from build123d import *

# Parameters (mm, degrees)
BASE_FLANGE1_DEPTH           = 50.8
CUT_EXTRUDE1_DEPTH           = 72.510156621
CUT_EXTRUDE1_DEPTH_BACK      = 72.510156621
SKETCH6_W                    = 21.9
SKETCH6_H                    = 58.896012785
SKETCH6_W_2                  = 19
F_7_0_7_DIAMETER_HOLE1_D     = 7
F_7_0_7_DIAMETER_HOLE1_DEPTH = 10
F_7_0_7_DIAMETER_HOLE1_TIP   = 2.103012167
CUT_EXTRUDE2_DEPTH           = 10
CHAMFER1_SIZE                = 0.5


# Sheet-metal steps are written as plain solids
with BuildPart() as part:
    # Sketch1 → Base-Flange1 (new, symmetric)
    with BuildSketch(Plane(origin=(0, 0, 0), x_dir=(0, 0, -1), z_dir=(1, 0, 0))):
        with BuildLine():
            Line((50, -4.5), (5.275314915, -4.5))
            ThreePointArc((5.275314915, -4.5), (3.603327521, -4.640767872), (1.978412548, -5.059108369))
            Line((1.978412548, -5.059108369), (0.835379329, -5.458272884))
            ThreePointArc((0.835379329, -5.458272884), (-0.371159142, -5.680341687), (-1.588253888, -5.526296191))
            ThreePointArc((-1.588253888, -5.526296191), (-2.687165368, 5.083467546), (5.460998077, -1.8))
            Line((5.460998077, -1.8), (3.086651087, -1.017391304))
            ThreePointArc((3.086651087, -1.017391304), (-1.518832599, 2.873264265), (-0.897708719, -3.123558716))
            ThreePointArc((-0.897708719, -3.123558716), (-0.44129819, -3.181325777), (0.011153737, -3.098049977))
            Line((0.011153737, -3.098049977), (1.154186957, -2.698885462))
            ThreePointArc((1.154186957, -2.698885462), (3.185330673, -2.17595984), (5.275314915, -2))
            Line((5.275314915, -2), (50, -2))
            Line((50, -2), (50, -4.5))
        make_face()
    extrude(amount=BASE_FLANGE1_DEPTH, both=True)

    # Sketch6 → Cut-Extrude1 (cut, two sides: drawn at the far end of the back side and taken through both)
    with BuildSketch(Plane(origin=(0, 0, 0), x_dir=(1, 0, 0), z_dir=(0, 1, 0)).offset(-CUT_EXTRUDE1_DEPTH_BACK)):
        with Locations((-39.85, -22.948006393)):
            Rectangle(SKETCH6_W, SKETCH6_H)
        with Locations((39.85, -22.948006393)):
            Rectangle(SKETCH6_W, SKETCH6_H)
        with Locations((0, -22.948006393)):
            Rectangle(SKETCH6_W_2, SKETCH6_H)
    extrude(amount=CUT_EXTRUDE1_DEPTH + CUT_EXTRUDE1_DEPTH_BACK, mode=Mode.SUBTRACT)

    # Ø7.0 (7) Diameter Hole1
    with Locations(Plane(origin=(0, -2, 0), x_dir=(1, 0, 0), z_dir=(0, 1, 0))):
        with Locations((37.8, 27.2), (-37.8, 27.2), (12.8, 36.2)):
            Hole(F_7_0_7_DIAMETER_HOLE1_D / 2, depth=F_7_0_7_DIAMETER_HOLE1_DEPTH)
            with Locations((0, 0, -(F_7_0_7_DIAMETER_HOLE1_DEPTH + F_7_0_7_DIAMETER_HOLE1_TIP / 2))):  # 118° drill point
                Cone(0, F_7_0_7_DIAMETER_HOLE1_D / 2, F_7_0_7_DIAMETER_HOLE1_TIP, mode=Mode.SUBTRACT)

    # Sketch9 → Cut-Extrude2 (cut)
    with BuildSketch(Plane(origin=(0, -2, 0), x_dir=(1, 0, 0), z_dir=(0, 1, 0))):
        with BuildLine():
            Line((-9.7, 37.9), (-9.7, 31.9))
            ThreePointArc((-9.7, 31.9), (-12.8, 28.8), (-15.9, 31.9))
            Line((-15.9, 31.9), (-15.9, 37.9))
            ThreePointArc((-15.9, 37.9), (-12.8, 41), (-9.7, 37.9))
        make_face()
    extrude(amount=-CUT_EXTRUDE2_DEPTH, mode=Mode.SUBTRACT)

    # Chamfer1
    chamfer1_edges = [part.edges().sort_by_distance(p)[0] for p in [
        (16.3, -2, -36.2),
        (-34.3, -2, -27.2),
        (41.3, -2, -27.2),
        (-12.8, -2, -41),
        (-15.9, -2, -34.9),
        (-12.8, -2, -28.8),
        (-9.7, -2, -34.9),
    ]]
    chamfer(chamfer1_edges, length=CHAMFER1_SIZE)


solid = part.part
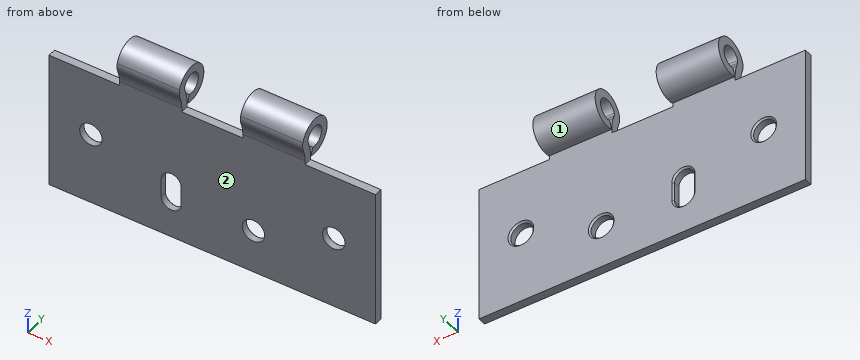
Verification items for the finished model (mm, model axes). Face numbers are marked on the shaded views. A direction names the side the tool comes from. Give positions to 0.01 mm unless a question says otherwise; leave off trailing zeros. Write each loop counter-clockwise with the first axis right and the second up, starting at its lowest first coordinate (ties: lowest second). Pieces come first, ordered by that corner, then holes. Notation, with made-up numbers: M 56.25,-4 L 115.25,-4 A11 ccw 115.25,6 Z; hole C -33,19.25 d11. An arc over 180 degrees is marked long. Write item = value, one per line.
(1) Go/stop test with flat-tipped pins: pin 1 Ø3 at (x, y) = (40.5, -3) entering from +Z; pin 2 Ø6 at (x, z) = (7, -40.5) entering from +Y; pin 3 Ø3.5 at (y, z) = (-2.5, -1) entering from -X. Record where each tip stops, or that it passes through.
Found:
pin_1 = -6.5
pin_2 = -2
pin_3 = -28.9
(2) Material ranges on line 1 (X direction, y = -4, z = -27.2); line 2 (X direction, y = -3.4, z = -36.2); line 3 (Z direction, x = 21, y = 0), recorded low to high.
Found:
line_1 = -50.8 to -41.3, -34.3 to 34.3, 41.3 to 50.8
line_2 = -50.8 to -15.9, -9.7 to 9.3, 16.3 to 50.8
line_3 = -5.75 to -3.25, 3.25 to 5.75
(3) Sectioned sample at D-D (x = 19). Record the cut outline in (y, z).
Found:
outline = M -5.53,1.59 A4 ccw -5.46,-0.84 L -5.06,-1.98 A10 cw -4.5,-5.28 L -4.5,-50 L -2,-50 L -2,-5.28 A12.5 ccw -2.7,-1.15 L -3.1,-0.01 A1.5 cw -3.12,0.9 A3.25 cw long -1.02,-3.09 L -1.8,-5.46 A5.75 ccw long Z
(4) Sectioned sample at A-A (x = -37.8). Record the cut outline in (y, z).
Found:
outline = M -4.5,-50 L -2,-50 L -2,-31.2 L -2.5,-30.7 L -4.5,-30.7 Z; M -4.5,-23.7 L -2.5,-23.7 L -2,-23.2 L -2,-6.5 L -4.5,-6.5 Z
(5) Sectioned sample at B-B (y = 0). Record the cut outline in (x, z).
Found:
outline = M -28.9,-5.75 L -9.5,-5.75 L -9.5,-3.25 L -28.9,-3.25 Z; M -28.9,3.25 L -9.5,3.25 L -9.5,5.75 L -28.9,5.75 Z; M 9.5,-5.75 L 28.9,-5.75 L 28.9,-3.25 L 9.5,-3.25 Z; M 9.5,3.25 L 28.9,3.25 L 28.9,5.75 L 9.5,5.75 Z
(6) Sectioned sample at C-C (z = -36.2). Record the cut outline in (x, y), then the cut area to 4 significant figures.
Found:
outline = M -50.8,-4.5 L -15.9,-4.5 L -15.9,-2.5 L -16.4,-2 L -50.8,-2 Z; M -9.7,-4.5 L 9.3,-4.5 L 9.3,-2.5 L 8.8,-2 L -9.2,-2 L -9.7,-2.5 Z; M 16.3,-4.5 L 50.8,-4.5 L 50.8,-2 L 16.8,-2 L 16.3,-2.5 Z
area = 220.5 mm2
(7) Access from +Z, -Z, +X, -X, +Y, -Y to the whole of each face (thin tool, end or side, straight path). Record for the marked faces 1 and 2.
Found:
face_1 = +X, -X
face_2 = -Z, +X, -X, -Y
